Model file for the job. Use its own axes, mm. Round coordinates to 2 decimals unless told otherwise and drop trailing zeros. Loops run counter-clockwise (first coordinate to the right, second up) from the corner with the lowest first, then second, coordinate; pieces in that order, holes last. Notation, with made-up numbers: (72.25, 61) - (105.25, 61) arc R30 ccw to (105.25, 96) - close; hole circle Ø3 at (21.25, -19). An arc over 180 degrees is marked (long way). Answer as a JSON object with one key per item and string values.
from build123d import *

# Parameters (mm, degrees)
BOSS_EXTRUDE1_DEPTH = 28.83
SKETCH2_R           = 5.475
CUT_EXTRUDE1_DEPTH  = 82
SKETCH3_R           = 4
CUT_EXTRUDE4_DEPTH  = 29.83


with BuildPart() as part:
    # Sketch1 → Boss-Extrude1 (new body)
    with BuildSketch(Plane(origin=(0, 0, 0), x_dir=(1, 0, 0), z_dir=(0, 1, 0))):
        Polygon((5.97883519, 18.175658977), (-12.75116481, 14.265652648), (-18.73, -3.910006329), (-5.97883519, -18.175658977), (12.75116481, -14.265652648), (18.73, 3.910006329), align=None)
    extrude(amount=BOSS_EXTRUDE1_DEPTH)

    # Sketch2 → Cut-Extrude1 (cut)
    with BuildSketch(Plane(origin=(3.38616481, 0, 16.220655813), x_dir=(0.97889766, 0, -0.204351097), z_dir=(0.204351097, 0, 0.97889766))):
        with Locations((0, 14.415)):
            Circle(SKETCH2_R)
    extrude(amount=-CUT_EXTRUDE1_DEPTH, mode=Mode.SUBTRACT)

    # Sketch3 → Cut-Extrude4 (cut, through all)
    with BuildSketch(Plane(origin=(0, 28.83, 0), x_dir=(1, 0, 0), z_dir=(0, 1, 0))):
        with Locations((-5.253979625, -4.69620015)):
            Circle(SKETCH3_R)
    extrude(amount=-CUT_EXTRUDE4_DEPTH, mode=Mode.SUBTRACT)


solid = part.part
1) Two-plate mould, pull along Y, no slides. Class faces 1 (the cylindrical face through (5.16, 16.06, -0.84)), 2 (the flat face through (0, 28.83, 0)), 3 (the flat face through (15.7, 14.2, 5.3)): pulls with the +Y half, pulls with the -Y half, needs draft (parallel to the pull), parting line crosses it, or undercut.
Values follow:
{"face 1": "undercut", "face 2": "pulls with the +Y half", "face 3": "needs draft"}
2) Slice it at A-A on y = 10.5. List the corners of the cut face in (x, z), then the cut area to 3 significant figures.
Values follow:
{"outline": "(-18.73, 3.91) - (-12.75, -14.27) - (-7.13, -15.44) - (-3.7, 1.01) arc R4 cw (long way) to (-2.35, 7.45) - (-0.36, 17) - (-5.98, 18.18) - close; (0.36, -17) - (5.98, -18.18) - (18.73, -3.91) - (12.75, 14.27) - (7.13, 15.44) - close", "area": "655 mm²"}
3) Drop flat-ended pins along their axis: P1, Ø7, axis at x = -5.25, z = 4.7, coming from the +Y side; P2, Ø10, axis at y = 9.5, z = 14, coming from the +X side; P3, Ø5, axis at y = 6, z = -2, coming from the +X side; P4, Ø4, axis at y = 6.5, z = 6, coming from the +X side. Give the stop position or say it passes through.
Values follow:
{"P1": "through", "P2": "x = 14.48", "P3": "x = 18.73", "P4": "x = 16.13"}
4) Slice it at D-D on x = 16.5. List the corners of the cut face in (y, z), then the cut area to 3 significant figures.
Values follow:
{"outline": "(0, -6.4) - (28.83, -6.4) - (28.83, 2.87) - (0, 2.87) - close", "area": "267 mm²"}
5) Slice it at B-B on y = 7. List the corners of the cut face in (x, z), then the cut area to 3 significant figures.
Values follow:
{"outline": "(-18.73, 3.91) - (-12.75, -14.27) - (5.98, -18.18) - (18.73, -3.91) - (12.75, 14.27) - (-5.98, 18.18) - close; hole circle Ø8 at (-5.25, 4.7)", "area": "901 mm²"}
6) Probe probe 1 along Y at (x, z) = (-6.5, -15); probe 2 along X at (y, z) = (18.25, -5.5); probe 3 along X at (y, z) = (16.5, 11). List the from-to ranges inside material, lowest first.
Values follow:
{"probe 1": "0 to 10.04, 18.79 to 28.83", "probe 2": "-15.63 to -5.14, 2.84 to 17.31", "probe 3": "-12.39 to -2.88, 7.47 to 13.83"}
7) Slice it at C-C on x = 10. List the corners of the cut face in (y, z).
Values follow:
{"outline": "(0, -13.68) - (28.83, -13.68) - (28.83, 14.84) - (0, 14.84) - close"}
